Can you work these out from the model? Positions are in its coordinate system, mm. Face numbers are marked on the shaded views. Coordinates: 2 decimals unless noted, no trailing zeros. Order: outer loops, then holes, each group sorted by start corner. A loop starts at its lowest first (then second) coordinate and runs counter-clockwise, first axis right, second up. Notation, with made-up numbers: (-24.5, 28.25) -> (-12.5, 28.25) arc R12 ccw to (-12.5, 40.25) -> close; hole circle Ø4 at (14, 42.25). An arc over 180 degrees is marked (long way). Return JSON: item names as keys, results as strings. Group by question number.
1) If I drill on probe 1 along X at (y, z) = (42.5, 5); probe 2 along Y at (x, z) = (9, 3.5); probe 3 along Y at (x, z) = (15, 5.3), over which ranges is the centre line in solid material (lowest first)? Write a range as from..to.
2) For pin 1 (3.5 mm diameter, centred on x = 15, y = 88, fed in from -Z); pin 2 (5 mm diameter, centred on x = 16, y = 32, fed in from -Z), each with a flat end and sliding along its axis, tell me the tip position at first contact or that it passes through.
3) If we section it at A-A, the plane y = 50: Please give me the cut outline in (x, z), then the cut area to 3 significant figures.
4) Thinking about a two-plate mould opening in Y: for the marked faces 1, 2, 3 and 4, which applies, +Y half, -Y half, draft (parallel to the pull), parting line (faces both ways), or undercut?
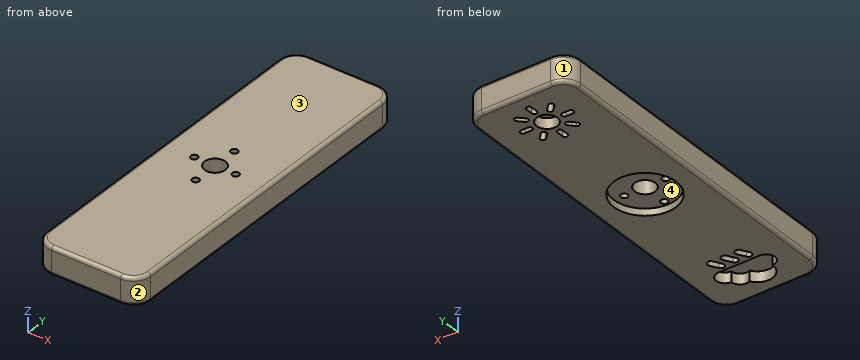
from build123d import *

# Parameters (mm, degrees)
EXTRUDE_1_DEPTH          = 8
SKETCH_2_R               = 3
CUT_EXTRUDE_1_DEPTH      = 3
CUT_EXTRUDE_2_DEPTH      = 3
PATTERN_CIRCULAR_1_COUNT = 8
CUT_EXTRUDE_3_DEPTH      = 3
CUT_EXTRUDE_4_DEPTH      = 3
PATTERN_LINEAR_2_COUNT   = 2
PATTERN_LINEAR_2_PITCH   = 4
PATTERN_LINEAR_4_COUNT   = 2
PATTERN_LINEAR_4_PITCH   = 4
SKETCH_14_R              = 9
CUT_EXTRUDE_7_DEPTH      = 2
SKETCH_15_R              = 3
CUT_EXTRUDE_8_DEPTH      = 7
SKETCH1_R                = 1
CUT_EXTRUDE1_DEPTH       = 7
CIRPATTERN1_COUNT        = 2
SKETCH2_R                = 1
CUT_EXTRUDE2_DEPTH       = 7
CIRPATTERN2_COUNT        = 2
FILLET1_R                = 1
FILLET2_R                = 1


with BuildPart() as part:
    # ｽｹｯﾁ1 → ﾎﾞｽ - 押し出し1 (new body)
    with BuildSketch(Plane.XY):
        with BuildLine():
            Line((5, 0), (25, 0))
            ThreePointArc((25, 0), (28.535533906, 1.464466094), (30, 5))
            Line((30, 5), (30, 95))
            ThreePointArc((30, 95), (28.535533906, 98.535533906), (25, 100))
            Line((25, 100), (5, 100))
            ThreePointArc((5, 100), (1.464466094, 98.535533906), (0, 95))
            Line((0, 95), (0, 5))
            ThreePointArc((0, 5), (1.464466094, 1.464466094), (5, 0))
        make_face()
    extrude(amount=EXTRUDE_1_DEPTH)

    # ｽｹｯﾁ2 → ｶｯﾄ - 押し出し1 (cut)
    with BuildSketch(Plane(origin=(0, 0, 0), x_dir=(-1, 0, 0), z_dir=(0, 0, -1))):
        with Locations((-15, 88)):
            Circle(SKETCH_2_R)
    extrude(amount=-CUT_EXTRUDE_1_DEPTH, mode=Mode.SUBTRACT)

    # ｽｹｯﾁ4 → ｶｯﾄ - 押し出し2 (cut)
    with BuildSketch(Plane(origin=(0, 0, 0), x_dir=(-1, 0, 0), z_dir=(0, 0, -1))):
        with BuildLine():
            Line((-14.25, 95), (-14.25, 93))
            ThreePointArc((-14.25, 93), (-15, 92.25), (-15.75, 93))
            Line((-15.75, 93), (-15.75, 95))
            ThreePointArc((-15.75, 95), (-15, 95.75), (-14.25, 95))
        make_face()
    cut_extrude_2 = extrude(amount=-CUT_EXTRUDE_2_DEPTH, mode=Mode.SUBTRACT)

    # 円形ﾊﾟﾀｰﾝ1: ｶｯﾄ - 押し出し2 ×8 about axis
    pattern_circular_1_axis = Axis((15, 88, 0), (0, 0, 1))
    for i in range(1, PATTERN_CIRCULAR_1_COUNT):
        add(cut_extrude_2.rotate(pattern_circular_1_axis, i * 360 / PATTERN_CIRCULAR_1_COUNT), mode=Mode.SUBTRACT)

    # ｽｹｯﾁ6 → ｶｯﾄ - 押し出し3 (cut)
    with BuildSketch(Plane(origin=(0, 0, 0), x_dir=(-1, 0, 0), z_dir=(0, 0, -1))):
        with BuildLine():
            Line((-9.000000044, 13.498973843), (-21, 13.5))
            ThreePointArc((-21, 13.5), (-23.5, 11), (-21, 8.5))
            ThreePointArc((-21, 8.5), (-19.822875656, 6.378679656), (-17.4, 6.255005568))
            ThreePointArc((-17.4, 6.255005568), (-12.337609323, 4.152719481), (-9.000000117, 8.501026157))
            ThreePointArc((-9.000000117, 8.501026157), (-6.501026157, 10.999999963), (-9.000000044, 13.498973843))
        make_face()
    extrude(amount=-CUT_EXTRUDE_3_DEPTH, mode=Mode.SUBTRACT)

    # ｽｹｯﾁ12 → ｶｯﾄ - 押し出し4 (cut)
    with BuildSketch(Plane(origin=(0, 0, 0), x_dir=(-1, 0, 0), z_dir=(0, 0, -1))):
        with BuildLine():
            Line((-15.258974596, 18.082531755), (-14.008974596, 15.917468245))
            ThreePointArc((-14.008974596, 15.917468245), (-14.375, 14.551442841), (-15.741025404, 14.917468245))
            Line((-15.741025404, 14.917468245), (-16.991025404, 17.082531755))
            ThreePointArc((-16.991025404, 17.082531755), (-16.625, 18.448557159), (-15.258974596, 18.082531755))
        make_face()
    cut_extrude_4 = extrude(amount=-CUT_EXTRUDE_4_DEPTH, mode=Mode.SUBTRACT)

    # 直線ﾊﾟﾀｰﾝ2: ｶｯﾄ - 押し出し4 ×2
    with Locations(*[(-i * PATTERN_LINEAR_2_PITCH, 0, 0) for i in range(1, PATTERN_LINEAR_2_COUNT)]):
        add(cut_extrude_4, mode=Mode.SUBTRACT)

    # 直線ﾊﾟﾀｰﾝ4: ｶｯﾄ - 押し出し4 ×2
    with Locations(*[(i * PATTERN_LINEAR_4_PITCH, 0, 0) for i in range(1, PATTERN_LINEAR_4_COUNT)]):
        add(cut_extrude_4, mode=Mode.SUBTRACT)

    # ｽｹｯﾁ14 → ｶｯﾄ - 押し出し7 (cut)
    with BuildSketch(Plane(origin=(0, 0, 0), x_dir=(-1, 0, 0), z_dir=(0, 0, -1))):
        with Locations((-15, 50)):
            Circle(SKETCH_14_R)
    extrude(amount=-CUT_EXTRUDE_7_DEPTH, mode=Mode.SUBTRACT)

    # ｽｹｯﾁ15 → ｶｯﾄ - 押し出し8 (cut, through all)
    with BuildSketch(Plane(origin=(0, 0, 2), x_dir=(-1, 0, 0), z_dir=(0, 0, -1))):
        with Locations((-15, 50)):
            Circle(SKETCH_15_R)
    extrude(amount=-CUT_EXTRUDE_8_DEPTH, mode=Mode.SUBTRACT)

    # Sketch1 → Cut-Extrude1 (cut, through all)
    with BuildSketch(Plane(origin=(0, 0, 2), x_dir=(-1, 0, 0), z_dir=(0, 0, -1))):
        with Locations((-15, 57.5)):
            Circle(SKETCH1_R)
    cut_extrude1 = extrude(amount=-CUT_EXTRUDE1_DEPTH, mode=Mode.SUBTRACT)

    # CirPattern1: Cut-Extrude1 ×2 about axis
    cirpattern1_axis = Axis((15, 50, 0), (0, 0, 1))
    for i in range(1, CIRPATTERN1_COUNT):
        add(cut_extrude1.rotate(cirpattern1_axis, i * 360 / CIRPATTERN1_COUNT), mode=Mode.SUBTRACT)

    # Sketch2 → Cut-Extrude2 (cut, through all)
    with BuildSketch(Plane(origin=(0, 0, 2), x_dir=(-1, 0, 0), z_dir=(0, 0, -1))):
        with Locations((-21, 50)):
            Circle(SKETCH2_R)
    cut_extrude2 = extrude(amount=-CUT_EXTRUDE2_DEPTH, mode=Mode.SUBTRACT)

    # CirPattern2: Cut-Extrude2 ×2 about axis
    cirpattern2_axis = Axis((15, 50, 0), (0, 0, 1))
    for i in range(1, CIRPATTERN2_COUNT):
        add(cut_extrude2.rotate(cirpattern2_axis, i * 360 / CIRPATTERN2_COUNT), mode=Mode.SUBTRACT)

    # Fillet1
    fillet1_edges = [part.edges().sort_by_distance(p)[0] for p in [
        (28.535533906, 98.535533906, 8),
        (15, 100, 8),
        (1.464466094, 98.535533906, 8),
        (0, 50, 8),
        (1.464466094, 1.464466094, 8),
        (15, 0, 8),
        (28.535533906, 1.464466094, 8),
        (30, 50, 8),
    ]]
    fillet(fillet1_edges, radius=FILLET1_R)

    # Fillet2
    fillet2_edges = [part.edges().sort_by_distance(p)[0] for p in [
        (15, 100, 0),
        (28.535533906, 98.535533906, 0),
        (30, 50, 0),
        (28.535533906, 1.464466094, 0),
        (15, 0, 0),
        (1.464466094, 1.464466094, 0),
        (0, 50, 0),
        (1.464466094, 98.535533906, 0),
    ]]
    fillet(fillet2_edges, radius=FILLET2_R)


solid = part.part
Result sheet:
{
 "1": {"probe 1": "x = 0..14, 16..30", "probe 2": "y = 0..49, 51..100", "probe 3": "y = 0..41.5, 43.5..47, 53..56.5, 58.5..100"},
 "2": {"pin 1": "stops at z = 3", "pin 2": "stops at z = 0"},
 "3": {"outline": "(0, 1) arc R1 ccw to (1, 0) -> (6, 0) -> (6, 2) -> (8, 2) -> (8, 8) -> (1, 8) arc R1 ccw to (0, 7) -> close; (10, 2) -> (12, 2) -> (12, 8) -> (10, 8) -> close; (18, 2) -> (20, 2) -> (20, 8) -> (18, 8) -> close; (22, 2) -> (24, 2) -> (24, 0) -> (29, 0) arc R1 ccw to (30, 1) -> (30, 7) arc R1 ccw to (29, 8) -> (22, 8) -> close", "area": "143 mm2"},
 "4": {"face 1": "+Y half", "face 2": "-Y half", "face 3": "draft", "face 4": "undercut"}
}
